For this review, take the finished solid that the model builds, in its own axes (mm). Face numbers are marked on the shaded views. A direction names the side the tool comes from. Round coordinates to 2 decimals unless told otherwise and drop trailing zeros. Loops run counter-clockwise (first coordinate to the right, second up) from the corner with the lowest first, then second, coordinate; pieces in that order, holes last.
1) Take a section at B-B (y = -1.75). State the section outline as (x, z) points, then the cut area to 3 significant figures.
2) Take a section at C-C (x = 9.5). State the section outline as (y, z) points, then the cut area to 3 significant figures.
3) Insertion check: pin 1 (5 mm diameter, centred on x = 4, y = -2, fed in from +Z); pin 2 (0.8 mm diameter, centred on x = 5.5, z = 2, fed in from +Y); pin 3 (1.3 mm diameter, centred on y = -4.5, z = 3, fed in from -X). Each pin has a flat end and moves straight along its axis. Give the tip position at first contact, or say it passes through.
4) Tool access review of the marked faces 1, 2 and 3: name each direction out of +Z, -Z, +X, -X, +Y, -Y from which nothing blocks a thin tool from reaching the whole face with its end or side.
5) Take a section at A-A (z = 2). State the section outline as (x, y) points, then the cut area to 3 significant figures.
6) Mouldability with a two-part tool opening along X and no side actions: class the marked faces 4, 5, 6 and 7 as pulls with the +X half, pulls with the -X half, needs draft (parallel to the pull), parting line crosses it, or undercut.
7) Wall thickness on L1, parallel to X at y = 0.75, z = 2.5; L2, parallel to Y at x = -4.25, z = 3.1; L3, parallel to Z at x = 6.75, y = 4: over which ranges is each line inside the solid? List them lowest first.
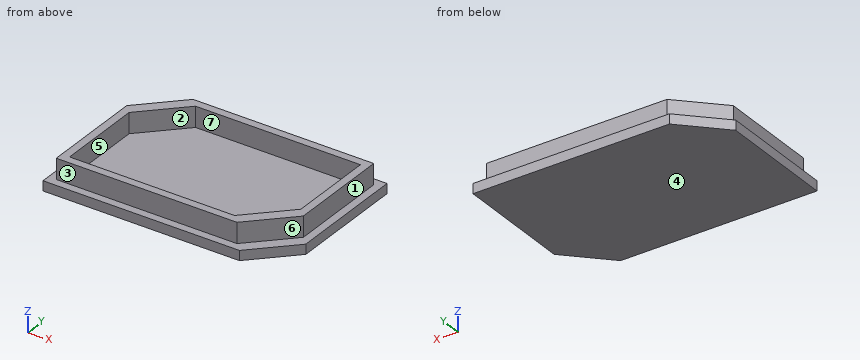
```python
from build123d import *

# Parameters (mm, degrees)
F0_W     = 30
F0_H     = 20
F1_DEPTH = 1.25
F2_W     = 28
F2_H     = 18
F3_DEPTH = 2.6
F4_W     = 26
F4_H     = 16
F5_DEPTH = 2.6
F6_SIZE  = 5
F7_SIZE  = 5


with BuildPart() as f1:
    # F0 (on Top) → F1 (new body)
    with BuildSketch(Plane.XY):
        Rectangle(F0_W, F0_H)
    extrude(amount=F1_DEPTH)

    # F2 (on face) → F3 (join)
    with BuildSketch(Plane.XY.offset(1.25)):
        Rectangle(F2_W, F2_H)
    extrude(amount=F3_DEPTH)

    # F4 (on face) → F5 (cut)
    with BuildSketch(Plane.XY.offset(3.85)):
        Rectangle(F4_W, F4_H)
    extrude(amount=-F5_DEPTH, mode=Mode.SUBTRACT)

    # F6
    f6_edges = [f1.edges().sort_by_distance(p)[0] for p in [
        (-13, 8, 2.55),
        (13, -8, 2.55),
        (-14, 9, 2.55),
        (14, -9, 2.55),
    ]]
    chamfer(f6_edges, length=F6_SIZE)

    # F7
    f7_edges = [f1.edges().sort_by_distance(p)[0] for p in [
        (15, -10, 0.625),
        (-15, 10, 0.625),
    ]]
    chamfer(f7_edges, length=F7_SIZE)


solid = f1.part
```
Response:
1. outline: (-15, 0) - (15, 0) - (15, 1.25) - (14, 1.25) - (14, 3.85) - (13, 3.85) - (13, 1.25) - (-13, 1.25) - (-13, 3.85) - (-14, 3.85) - (-14, 1.25) - (-15, 1.25) - close
1. area: 42.7 mm2
2. outline: (-10, 0) - (10, 0) - (10, 1.25) - (9, 1.25) - (9, 3.85) - (8, 3.85) - (8, 1.25) - (-6.5, 1.25) - (-6.5, 3.85) - (-8.5, 3.85) - (-8.5, 1.25) - (-10, 1.25) - close
2. area: 32.8 mm2
3. pin 1: stops at z = 1.25
3. pin 2: stops at y = 9
3. pin 3: stops at x = -14
4. face 1: +Z, +X, +Y, -Y
4. face 2: +Z
4. face 3: +Z, +X, -X, -Y
5. outline: (-14, -9) - (9, -9) - (14, -4) - (14, 9) - (-9, 9) - (-14, 4) - close; hole (-13, -8) - (8, -8) - (13, -3) - (13, 8) - (-8, 8) - (-13, 3) - close
5. area: 88.0 mm2
6. face 4: needs draft
6. face 5: undercut
6. face 6: pulls with the +X half
6. face 7: undercut
7. L1: x = -14 to -13, 13 to 14
7. L2: y = -9 to -8, 8 to 9
7. L3: z = 0 to 1.25
